Design review of the part built by this model. Coordinates are the model's own, in mm. A direction names the side the tool comes from. Give positions to 0.01 mm unless a question says otherwise; leave off trailing zeros. Order: outer loops, then holes, each group sorted by start corner. A loop starts at its lowest first (then second) coordinate and runs counter-clockwise, first axis right, second up.
```python
from build123d import *

# Parameters (mm, degrees)
F1_DEPTH    = 40
F2_R        = 2.4142135624
F3_R        = 10.2321597652
F4_T1_DEPTH = 40
F4_T3_DEPTH = 48.4497474683
F5_R        = 0.5


# Not quite as in the source:
# - a fillet or chamfer that OpenCascade refuses, or shapes differently, is made with other operations: its cross-section is extruded or revolved along the edge and cut away or added


with BuildPart() as f1:
    # F0 (on Right) → F1 (new body)
    with BuildSketch(Plane.YZ):
        with BuildLine():
            ThreePointArc((-25.4094946088, 3.7613025295), (-26.6631912182, 5.323376139), (-28.4595870608, 4.4374917638))
            ThreePointArc((-28.4595870608, 4.4374917638), (-27.6856838354, 2.3112100739), (-25.5594021496, 3.0851133107))
            ThreePointArc((-25.5594021496, 3.0851133107), (-25.4474209974, 3.4149991472), (-25.4094946088, 3.7613025295))
        make_face()
        with BuildLine():
            ThreePointArc((-16.0431703857, -1.3523784376), (-15.774850852, -0.6883818658), (-15.577323066, 0))
            Line((-15.577323066, 0), (-18.9433553042, 0))
            ThreePointArc((-18.9433553042, 0), (-23.7939353822, -1.7654667673), (-25.5594021496, 3.0851133107))
            ThreePointArc((-25.5594021496, 3.0851133107), (-27.6856838354, 2.3112100739), (-28.4595870608, 4.4374917638))
            ThreePointArc((-28.4595870608, 4.4374917638), (-25.1463138276, -4.6656516822), (-16.0431703857, -1.3523784376))
        make_face()
        with BuildLine():
            ThreePointArc((-15.4013787269, 1.5425566554), (-15.4524550708, 2.3775040298), (-15.604922411, 3.2))
            Line((-15.604922411, 3.2), (-17.4511707981, 3.2))
            Line((-17.4511707981, 3.2), (-18.9433553042, 0))
            Line((-18.9433553042, 0), (-15.577323066, 0))
            ThreePointArc((-15.577323066, 0), (-15.4455069504, 0.7662774779), (-15.4013787269, 1.5425566554))
        make_face()
        with BuildLine():
            Line((-15.4125459635, 0), (-13.9203614574, 3.2))
            Line((-13.9203614574, 3.2), (-15.604922411, 3.2))
            ThreePointArc((-15.604922411, 3.2), (-15.4524550708, 2.3775040298), (-15.4013787269, 1.5425566554))
            ThreePointArc((-15.4013787269, 1.5425566554), (-15.4455069504, 0.7662774779), (-15.577323066, 0))
            Line((-15.577323066, 0), (-15.4125459635, 0))
        make_face()
        Polygon((-2.0386248346, 0), (0, 0), (0, 3.2), (-13.9203614574, 3.2), (-15.4125459635, 0), align=None)
        with BuildLine():
            Line((-15.604922411, 3.2), (-13.9203614574, 3.2))
            Line((-13.9203614574, 3.2), (-2.3315382908, 28.0523114815))
            Line((-2.3315382908, 28.0523114815), (0, 33.0523114815))
            Line((0, 33.0523114815), (7, 33.0523114815))
            Line((7, 33.0523114815), (7, 0))
            Line((7, 0), (10.2, 0))
            Line((10.2, 0), (10.2, 36.2523114815))
            Line((10.2, 36.2523114815), (-2.0386248346, 36.2523114815))
            Line((-2.0386248346, 36.2523114815), (-16.4936271239, 5.253459036))
            ThreePointArc((-16.4936271239, 5.253459036), (-15.9648640306, 4.2632611548), (-15.604922411, 3.2))
        make_face()
        with BuildLine():
            Line((-16.0431703857, -1.3523784376), (-15.4125459635, 0))
            Line((-15.4125459635, 0), (-15.577323066, 0))
            ThreePointArc((-15.577323066, 0), (-15.774850852, -0.6883818658), (-16.0431703857, -1.3523784376))
        make_face()
        with BuildLine():
            Line((-17.4511707981, 3.2), (-15.604922411, 3.2))
            ThreePointArc((-15.604922411, 3.2), (-15.9648640306, 4.2632611548), (-16.4936271239, 5.253459036))
            Line((-16.4936271239, 5.253459036), (-17.4511707981, 3.2))
        make_face()
        Polygon((-2.3315382908, 28.0523114815), (0, 28.0523114815), (0, 33.0523114815), align=None)
    extrude(amount=F1_DEPTH)

    # F2
    f2_edges = [f1.edges().sort_by_distance(p)[0] for p in [
        (20, -2.038625, 36.252311),
        (20, 10.2, 36.252311),
    ]]
    fillet(f2_edges, radius=F2_R)

    # F3
    f3_edges = [f1.edges().sort_by_distance(p)[0] for p in [
        (20, -15.412546, 0),
    ]]
    fillet(f3_edges, radius=F3_R)

    # F4: fillet of radius 1.6899494937 on 6 edges, made by hand

    # F4_s2 → F4_t1 (join)
    with BuildSketch(Plane.YZ):
        with BuildLine():
            ThreePointArc((-11.2676721112, 3.2), (-12.692961058, 3.9819402926), (-12.799286497, 5.6041530111))
            Line((-12.799286497, 5.6041530111), (-13.9203614574, 3.2))
            Line((-13.9203614574, 3.2), (-11.2676721112, 3.2))
        make_face()
        with BuildLine():
            ThreePointArc((-2.7865361119, 27.0765655052), (-2.1629309272, 27.7876509346), (-1.2549217261, 28.0523114815))
            Line((-1.2549217261, 28.0523114815), (-2.3315382908, 28.0523114815))
            Line((-2.3315382908, 28.0523114815), (-2.7865361119, 27.0765655052))
        make_face()
    extrude(amount=F4_T1_DEPTH)

    # F4_s4 → F4_t3 (cut)
    with BuildSketch(Plane.YZ.offset(-4.2248737342)):
        with BuildLine():
            ThreePointArc((8.6899494937, 0), (7.4949747468, 0.4949747468), (7, 1.6899494937))
            Line((7, 1.6899494937), (7, 0))
            Line((7, 0), (8.6899494937, 0))
        make_face()
        with BuildLine():
            ThreePointArc((0, 1.5100505063), (-0.4949747468, 2.7050252532), (-1.6899494937, 3.2))
            Line((-1.6899494937, 3.2), (0, 3.2))
            Line((0, 3.2), (0, 1.5100505063))
        make_face()
        with BuildLine():
            ThreePointArc((-1.6899494937, 0), (-0.4949747468, 0.4949747468), (0, 1.6899494937))
            Line((0, 1.6899494937), (0, 0))
            Line((0, 0), (-1.6899494937, 0))
        make_face()
        with BuildLine():
            ThreePointArc((10.2, 1.6899494937), (9.7050252532, 0.4949747468), (8.5100505063, 0))
            Line((8.5100505063, 0), (10.2, 0))
            Line((10.2, 0), (10.2, 1.6899494937))
        make_face()
    extrude(amount=F4_T3_DEPTH, mode=Mode.SUBTRACT)

    # F5
    f5_edges = [f1.edges().sort_by_distance(p)[0] for p in [
        (20, 0, 28.052311),
    ]]
    fillet(f5_edges, radius=F5_R)


solid = f1.part
```
1. Draft analysis for pull direction Y (two halves, no side actions). For faces 1 (the face through (20, 10.2, 18)), 2 (the face through (0, -8, 17)), 3 (the face through (20, 0, 31)), state which applies: pulls with the +Y half, pulls with the -Y half, needs draft (parallel to the pull), parting line crosses it, or undercut.
Recorded:
face 1: pulls with the +Y half
face 2: needs draft
face 3: undercut
2. Take a section at B-B (y = -21.5). State the section outline as (x, z) points, then the cut area to 3 significant figures.
Recorded:
outline: (0, -5.27) - (40, -5.27) - (40, -2.03) - (0, -2.03) - close
area: 129 mm2
3. Take a section at C-C (z = 31). State the section outline as (x, y) points, then the cut area to 3 significant figures.
Recorded:
outline: (0, -4.49) - (40, -4.49) - (40, 0) - (0, 0) - close; (0, 7) - (40, 7) - (40, 10.2) - (0, 10.2) - close
area: 308 mm2
4. For line 1 along Y through (x, z) = (12.5, 0.5); line 2 along Z through (x, y) = (12, 3); line 3 along Z through (x, y) = (15, -9.5), list the stretches that pass through material, from the lowest coordinate up.
Recorded:
line 1: y = -29.02 to -25.75, -18.71 to -0.49, 7.49 to 9.71
line 2: z = 33.05 to 36.25
line 3: z = 0 to 3.2, 12.68 to 20.25
5. Machinability: for faces 4 (the face through (19.72, -7.863, 16.19)), 5 (the face through (20, -6, 0)), 6 (the face through (20.28, 9.51, 35.53)), 7 (the face through (19.72, 7.48, 0.51)), which of the approach directions +Z, -Z, +X, -X, +Y, -Y give a long, thin tool a straight path to every point of the face, cutting with its end or side? Answer none if there is none.
Recorded:
face 4: +X, -X
face 5: -Z, +X, -X, +Y
face 6: +Z, +X, -X, +Y
face 7: -Z, +X, -X
6. For pin 1 (3.5 mm diameter, centred on x = 19, y = 2, fed in from -Z); pin 2 (0.8 mm diameter, centred on x = 10, y = -1, fed in from -Z); pin 3 (1 mm diameter, centred on x = 10.5, y = -24, fed in from -Z), all flat-tipped, find the tip position at first contact; note any pin that passes through.
Recorded:
pin 1: stops at z = 33.05
pin 2: stops at z = 0.03
pin 3: stops at z = -5.19
7. Take a section at A-A (z = 22). State the section outline as (x, y) points, then the cut area to 3 significant figures.
Recorded:
outline: (0, -8.68) - (40, -8.68) - (40, -5.15) - (0, -5.15) - close; (0, 7) - (40, 7) - (40, 10.2) - (0, 10.2) - close
area: 269 mm2
